For this review, take the finished solid that the model builds, in its own axes (mm). A direction names the side the tool comes from. Give positions to 0.01 mm unless a question says otherwise; leave off trailing zeros. Order: outer loops, then holes, each group sorted by start corner. A loop starts at its lowest first (then second) coordinate and runs counter-clockwise, first axis right, second up. Notation, with made-up numbers: (25.5, 27.5) -> (75.5, 27.5) arc R15 ccw to (75.5, 44.5) -> close; hole circle Ø9 at (48, 36.5). An arc over 180 degrees is marked (long way). Return JSON: item names as keys, results as strings. Group by question number.
1) Add section D-D (z = 4). Give the boundary of the cut face in (x, y), then the cut area to 3 significant figures.
2) Insertion check: P1, Ø3, axis at x = 11, y = 4, coming from the +Z side; P2, Ø7.5, axis at y = 6, z = 8.5, coming from the +X side; P3, Ø4.5, axis at y = 6, z = 8, coming from the -X side. Each pin has a flat end and moves straight along its axis. Give the tip position at first contact, or say it passes through.
3) Add section B-B (z = -10.5). Give the boundary of the cut face in (x, y), then the cut area to 3 significant figures.
4) For faces 4 (the face through (-17.5, 7, -7)), 5 (the face through (-11.7, 7.395, 8.046)), list the 3-axis set-ups (+Z, -Z, +X, -X, +Y, -Y) from which the entire face can be reached by the end or side of a thin tool; tool diameter is ignored.
5) Add section C-C (y = 2.25). Give the boundary of the cut face in (x, z), then the cut area to 3 significant figures.
6) To check wall thickness, follow line 1 along X through (y, z) = (0.75, -4.5); line 2 along Z through (x, y) = (-2, 12.25); line 3 along Z through (x, y) = (3.5, 6.5). State the ranges of each line that lie inside material, in increasing order.
7) The part is to be moulded in two halves that separate along X. For faces 1 (the face through (2.75, 7, -7)), 2 (the face through (17.5, 7, -8)), 3 (the face through (0, 15, 1)), say which applies: released by +X, released by -X, zero draft, split by the parting line, or undercut.
8) Add section A-A (x = 1). Give the boundary of the cut face in (y, z), then the cut area to 3 significant figures.
from build123d import *

# Parameters (mm, degrees)
SFIVEBASETP1_W     = 12.75
SFIVEBASETP1_H     = 13
SFIVEBASETP1_W_2   = 5.5
FFIVEBASETP1_DEPTH = 15


with BuildPart() as part:
    # SFiveBaseTP1 → FFiveBaseTP1 (new body)
    with BuildSketch(Plane(origin=(0, 0, 0), x_dir=(1, 0, 0), z_dir=(0, 1, 0))):
        Polygon((-17.5, 15), (17.5, 15), (17.5, 0), (7.5, -17.320508076), (-7.5, -17.320508076), (-17.5, 0), align=None)
        Polygon((-16.345299462, 0), (-6.922649731, -16.320508076), (-0.5, -16.320508076), (-0.5, 0), align=None, mode=Mode.SUBTRACT)
        with Locations((-10.125, 7.5)):
            Rectangle(SFIVEBASETP1_W, SFIVEBASETP1_H, mode=Mode.SUBTRACT)
        with Locations((10.125, 7.5)):
            Rectangle(SFIVEBASETP1_W, SFIVEBASETP1_H, mode=Mode.SUBTRACT)
        Polygon((0.5, 0), (0.5, -16.320508076), (6.922649731, -16.320508076), (16.345299462, 0), align=None, mode=Mode.SUBTRACT)
        with Locations((0, 7.5)):
            Rectangle(SFIVEBASETP1_W_2, SFIVEBASETP1_H, mode=Mode.SUBTRACT)
    extrude(amount=FFIVEBASETP1_DEPTH)


solid = part.part
Evaluation:
{
 "1": {"outline": "(-15.19, 0) -> (-14.04, 0) -> (-14.04, 15) -> (-15.19, 15) -> close; (-0.5, 0) -> (0.5, 0) -> (0.5, 15) -> (-0.5, 15) -> close; (14.04, 0) -> (15.19, 0) -> (15.19, 15) -> (14.04, 15) -> close", "area": "49.6 mm^2"},
 "2": {"P1": "z = 13.86", "P2": "x = 14.76", "P3": "x = -14.18"},
 "3": {"outline": "(-17.5, 0) -> (-16.5, 0) -> (-16.5, 15) -> (-17.5, 15) -> close; (-3.75, 0) -> (-2.75, 0) -> (-2.75, 15) -> (-3.75, 15) -> close; (2.75, 0) -> (3.75, 0) -> (3.75, 15) -> (2.75, 15) -> close; (16.5, 0) -> (17.5, 0) -> (17.5, 15) -> (16.5, 15) -> close", "area": "60.0 mm^2"},
 "4": {"face 4": "+Z, -Z, -X, +Y, -Y", "face 5": "+Y, -Y"},
 "5": {"outline": "(-17.5, -15) -> (17.5, -15) -> (17.5, 0) -> (7.5, 17.32) -> (-7.5, 17.32) -> (-17.5, 0) -> close; hole (-16.5, -14) -> (-3.75, -14) -> (-3.75, -1) -> (-16.5, -1) -> close; hole (-16.35, 0) -> (-0.5, 0) -> (-0.5, 16.32) -> (-6.92, 16.32) -> close; hole (-2.75, -14) -> (2.75, -14) -> (2.75, -1) -> (-2.75, -1) -> close; hole (0.5, 0) -> (16.35, 0) -> (6.92, 16.32) -> (0.5, 16.32) -> close; hole (3.75, -14) -> (16.5, -14) -> (16.5, -1) -> (3.75, -1) -> close", "area": "192 mm^2"},
 "6": {"line 1": "-17.5 to -16.5, -3.75 to -2.75, 2.75 to 3.75, 16.5 to 17.5", "line 2": "-15 to -14, -1 to 0, 16.32 to 17.32", "line 3": "-15 to 0, 16.32 to 17.32"},
 "7": {"face 1": "undercut", "face 2": "released by +X", "face 3": "zero draft"},
 "8": {"outline": "(0, -15) -> (15, -15) -> (15, -14) -> (0, -14) -> close; (0, -1) -> (15, -1) -> (15, 0) -> (0, 0) -> close; (0, 16.32) -> (15, 16.32) -> (15, 17.32) -> (0, 17.32) -> close", "area": "45.0 mm^2"}
}
